from build123d import *

# Parameters (mm, degrees)
SKETCH2_R           = 5
BOSS_EXTRUDE1_DEPTH = 7.5946
SKETCH3_R           = 0.9525
CUT_EXTRUDE1_DEPTH  = 2.54
FILLET1_R           = 0.127
SKETCH4_R           = 0.35
BOSS_EXTRUDE2_DEPTH = 5.5
SKETCH7_R           = 0.3556
BOSS_EXTRUDE3_DEPTH = 4.5
SKETCH6_R           = 1.143
CUT_EXTRUDE3_DEPTH  = 0.0762


with BuildPart() as part:
    # Sketch2 → Boss-Extrude1 (new body)
    with BuildSketch(Plane.XY):
        Circle(SKETCH2_R)
    extrude(amount=BOSS_EXTRUDE1_DEPTH)

    # Sketch3 → Cut-Extrude1 (cut)
    with BuildSketch(Plane.XY.offset(7.5946)):
        Circle(SKETCH3_R)
    extrude(amount=-CUT_EXTRUDE1_DEPTH, mode=Mode.SUBTRACT)

    # Fillet1
    fillet1_edges = [part.edges().sort_by_distance(p)[0] for p in [
        (-5, 0, 0),
        (-5, 0, 7.5946),
        (-0.9525, 0, 7.5946),
    ]]
    fillet(fillet1_edges, radius=FILLET1_R)

    # Sketch4 → Boss-Extrude2 (add)
    with BuildSketch(Plane(origin=(0, 0, 0), x_dir=(-1, 0, 0), z_dir=(0, 0, -1))):
        with Locations(Location((3.81, 0, 0), (0, 0, 180))):
            Circle(SKETCH4_R)
    extrude(amount=BOSS_EXTRUDE2_DEPTH)

    # Sketch7 → Boss-Extrude3 (add)
    with BuildSketch(Plane(origin=(0, 0, 0), x_dir=(-1, 0, 0), z_dir=(0, 0, -1))):
        with Locations(Location((-3.81, 0, 0), (0, 0, 180))):
            Circle(SKETCH7_R)
    extrude(amount=BOSS_EXTRUDE3_DEPTH)

    # Sketch6 → Cut-Extrude3 (cut)
    with BuildSketch(Plane.XY.offset(7.5946)):
        with Locations((-3.832516077, 0)):
            Circle(SKETCH6_R)
        Polygon((-3.912034188, 0.09834359), (-3.912034188, 0.722488889), (-3.722076923, 0.722488889), (-3.722076923, 0.09834359), (-3.097931624, 0.09834359), (-3.097931624, -0.091613675), (-3.722076923, -0.091613675), (-3.722076923, -0.715758974), (-3.912034188, -0.715758974), (-3.912034188, -0.091613675), (-4.536179487, -0.091613675), (-4.536179487, 0.09834359), align=None, mode=Mode.SUBTRACT)
    extrude(amount=-CUT_EXTRUDE3_DEPTH, mode=Mode.SUBTRACT)


solid = part.part
Read the model definition and answer for the solid it produces. Units are mm, in the model's axes. Round coordinates to 2 decimals unless told otherwise and drop trailing zeros. Loops run counter-clockwise (first coordinate to the right, second up) from the corner with the lowest first, then second, coordinate; pieces in that order, holes last. Notation, with made-up numbers: (-32.75, 77.25) - (7.25, 77.25) arc R24 ccw to (7.25, 101.25) - close; hole circle Ø5 at (79.5, 18.5). An arc over 180 degrees is marked (long way). One line per question, with ' | ' between items. Start each with the question number.
Q1. Section C-C on z = 5.75 is taken. Give the vertices of the cut face in (x, y) (1 decimal), plus the area to 3 significant figures.
Q2. Find the intervals of material crossed by L1, parallel to Y at x = 0, z = 6.8; L2, parallel to Z at x = -3.75, y = 3; L3, parallel to X at y = 0.5, z = 5.5, in increasing order.
Q3. Flat-ended cylindrical pins translate along their axes: pin 1 (0.8 mm diameter, centred on x = 4, y = 0, fed in from -Z); pin 2 (1.5 mm diameter, centred on x = -2, z = 4, fed in from -Y); pin 3 (2 mm diameter, centred on y = 0.5, z = -2, fed in from +X). Find the tip coordinate at first contact, or state that the pin passes through.
Q4. Section B-B on x = 0 is taken. Give the vertices of the cut face in (y, z), plus the area to 3 significant figures.
Q5. For a pull along X with two mould halves and no side action, classify faces 1 (the flat face through (1, -1, 7.595)), 2 (the cylindrical face through (-1.08, -4.88, 3.75)), 3 (the cylindrical face through (-0.21, -0.93, 6.28)) as +X half, -X half, draft (parallel to the pull), parting line (faces both ways), or undercut.
Q6. Section A-A on z = -4 is taken. Give the vertices of the cut face in (x, y).
Established:
1) outline: circle Ø10 at (0, 0); hole circle Ø1.9 at (0, 0) | area: 75.7 mm²
2) L1: -5 to -0.95, 0.95 to 5 | L2: 0 to 7.59 | L3: -4.97 to -0.81, 0.81 to 4.97
3) pin 1: z = -4.5 | pin 2: y = -4.84 | pin 3: x = 4.17
4) outline: (-5, 0.13) arc R0.13 ccw to (-4.87, 0) - (4.87, 0) arc R0.13 ccw to (5, 0.13) - (5, 7.47) arc R0.13 ccw to (4.87, 7.59) - (1.08, 7.59) arc R0.13 ccw to (0.95, 7.47) - (0.95, 5.05) - (-0.95, 5.05) - (-0.95, 7.47) arc R0.13 ccw to (-1.08, 7.59) - (-4.87, 7.59) arc R0.13 ccw to (-5, 7.47) - close | area: 71.1 mm²
5) face 1: draft | face 2: parting line | face 3: undercut
6) outline: circle Ø0.7 at (-3.81, 0); circle Ø0.71 at (3.81, 0)
